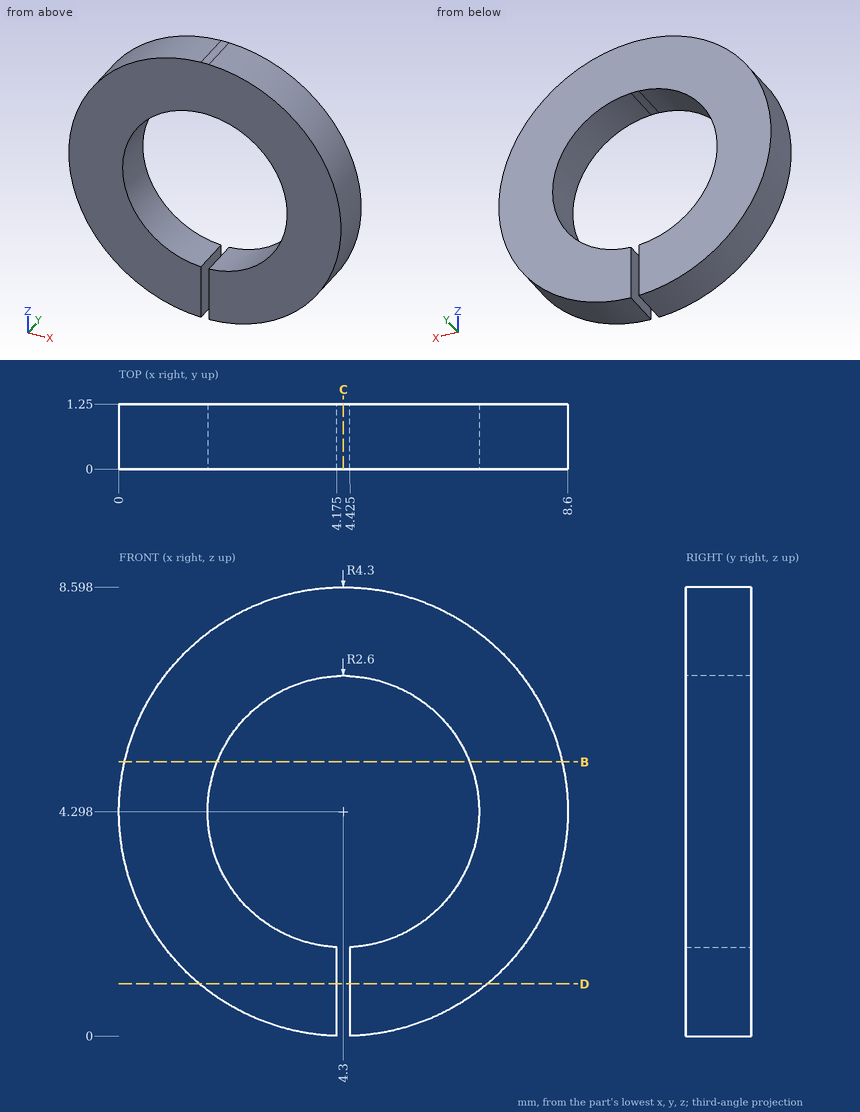
Job drawing, mm, ordinate dimensions from the low corner. One solid piece. Coordinates: 2 decimals unless noted, no trailing zeros. Loops run counter-clockwise (first coordinate to the right, second up) from the corner with the lowest first, then second, coordinate; pieces in that order, holes last. Notation, with made-up numbers: (4.25, 2.5) - (25.25, 2.5) arc R24 ccw to (25.25, 32.5) - close; hole circle Ø1 at (44.25, 40.25). An arc over 180 degrees is marked (long way). Write item = value, one per line. Start each with the question number.
Q1. Cut at B-B, the plane z = 5.25. List the corners of the cut face in (x, y).
Q2. Cut at D-D, the plane z = 1. List the corners of the cut face in (x, y) (3 decimals).
Q3. Drill centre lines: L1, parallel to X at y = 0.85, z = 5.25; L2, parallel to Z at x = 4.75, y = 0.7 (1 decimal); L3, parallel to Z at x = 5.5, y = 1 (1 decimal). Where is each one in solid material? Low to high.
Q4. Cut at C-C, the plane x = 4.3. List the corners of the cut face in (y, z).
Q5. Flat gauge pin, fed straight in: pin 1 Ø0.6 at (y, z) = (0.5, 0.5) entering from +X. Where does the tip first touch, or does it go through?
Computed:
q1.outline = (0.11, 0) - (1.88, 0) - (1.88, 1.25) - (0.11, 1.25) - close; (6.72, 0) - (8.49, 0) - (8.49, 1.25) - (6.72, 1.25) - close
q2.outline = (1.541, 0) - (4.175, 0) - (4.175, 1.25) - (1.541, 1.25) - close; (4.425, 0) - (7.059, 0) - (7.059, 1.25) - (4.425, 1.25) - close
q3.L1 = 0.11 to 1.88, 6.72 to 8.49
q3.L2 = 0 to 1.7, 6.9 to 8.6
q3.L3 = 0.2 to 2, 6.6 to 8.4
q4.outline = (0, 6.9) - (1.25, 6.9) - (1.25, 8.6) - (0, 8.6) - close
q5.pin_1 = 6.8
